Print and shaded views of the part. All mm, measured from the part's lowest x, y and z. Round coordinates to 2 decimals unless told otherwise and drop trailing zeros. Loops run counter-clockwise (first coordinate to the right, second up) from the corner with the lowest first, then second, coordinate; pieces in that order, holes last. Notation, with made-up numbers: (87, -6.5) - (92, -6.5) arc R10 cw to (92, 6.5) - close; hole circle Ø2 at (-36, 3.5). An arc over 180 degrees is marked (long way). Use one line per item in the form item = value.
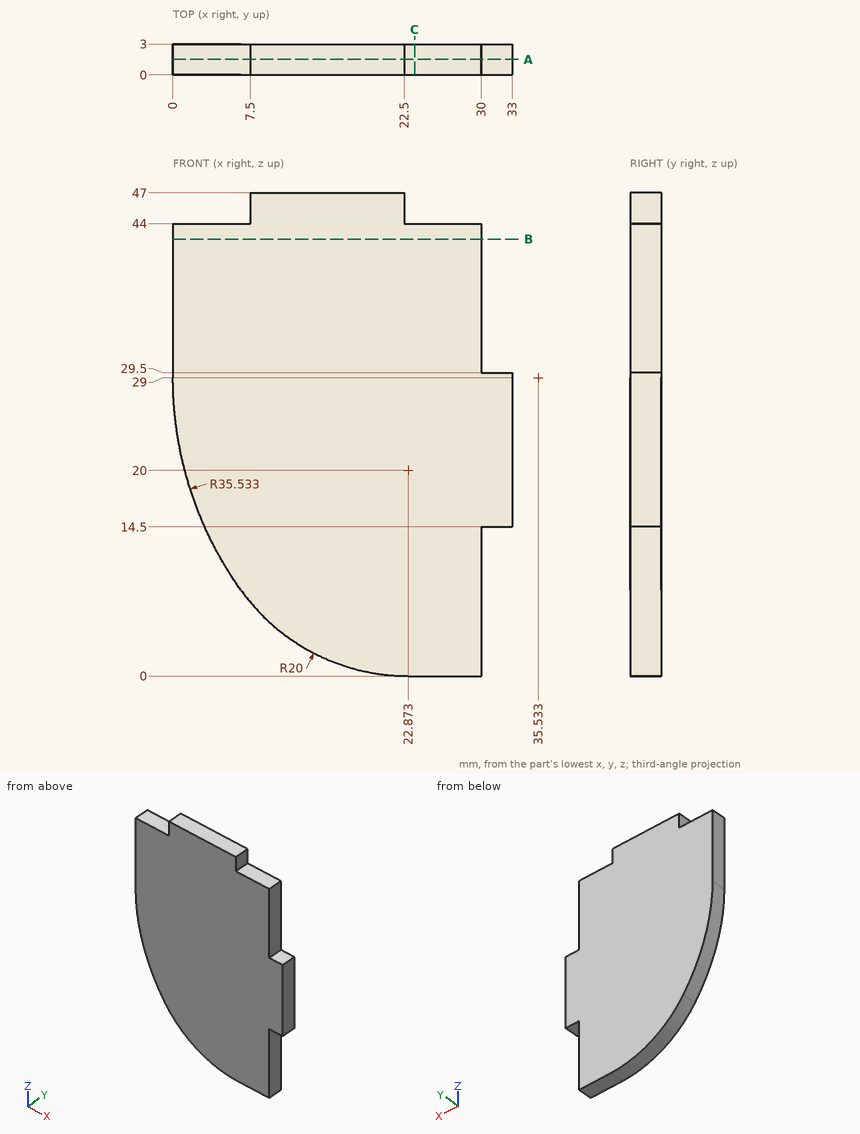
1) Slice it at A-A (y = 1.5). Write the cut outline in (x, z), plus the area to 3 significant figures.
Report:
outline = (0, 29) arc R35.53 ccw to (6.57, 8.41) arc R20 ccw to (22.87, 0) - (30, 0) - (30, 14.5) - (33, 14.5) - (33, 29.5) - (30, 29.5) - (30, 44) - (22.5, 44) - (22.5, 47) - (7.5, 47) - (7.5, 44) - (0, 44) - close
area = 1,270 mm^2
2) Flat gauge pins, fed straight in: pin 1 (0.9 mm diameter, centred on y = 1.5, z = 46, fed in from +X); pin 2 (0.9 mm diameter, centred on y = 1.5, z = 4, fed in from +X); pin 3 (0.9 mm diameter, centred on x = 27.5, y = 2, fed in from +Z). Where does each tip first touch, or does it go through?
Report:
pin_1 = 22.5
pin_2 = 30
pin_3 = 44
3) Drill centre lines: probe 1 along X at (y, z) = (0.35, 32.5); probe 2 along Z at (x, y) = (24, 2.1); probe 3 along X at (y, z) = (2.15, 21.5). Where is each one in solid material? Low to high.
Report:
probe_1 = 0 to 30
probe_2 = 0 to 44
probe_3 = 0.8 to 33
4) Slice it at C-C (x = 23.5). Write the cut outline in (y, z).
Report:
outline = (0, 0) - (3, 0) - (3, 44) - (0, 44) - close
5) Slice it at B-B (z = 42.5). Write the cut outline in (x, y), plus the area to 3 significant figures.
Report:
outline = (0, 0) - (30, 0) - (30, 3) - (0, 3) - close
area = 90.0 mm^2
